```python
from build123d import *

# Parameters (mm, degrees)
SKETCH1_R               = 2.7
BOSS_EXTRUDE1_DEPTH     = 35
CUT_EXTRUDE1_DEPTH      = 36.207669619
CUT_EXTRUDE1_DEPTH_BACK = 36.207669619
SKETCH2_W               = 9
SKETCH2_H               = 0.85
M3_TAPPED_HOLE1_D       = 2.5
M3_TAPPED_HOLE1_DEPTH   = 7.5
M3_TAPPED_HOLE1_TIP     = 0.751075774


with BuildPart() as part:
    # Sketch1 → Boss-Extrude1 (new body)
    with BuildSketch(Plane(origin=(0, 0, 0), x_dir=(0, 0, -1), z_dir=(1, 0, 0))):
        Circle(SKETCH1_R)
    extrude(amount=BOSS_EXTRUDE1_DEPTH)

    # Sketch2 → Cut-Extrude1 (cut, two sides: drawn at the far end of the back side and taken through both)
    with BuildSketch(Plane.XY.offset(-CUT_EXTRUDE1_DEPTH_BACK)):
        with Locations((30.5, 2.275)):
            Rectangle(SKETCH2_W, SKETCH2_H)
        with Locations((30.5, -2.275)):
            Rectangle(SKETCH2_W, SKETCH2_H)
        with Locations((4.5, -2.275)):
            Rectangle(SKETCH2_W, SKETCH2_H)
        with Locations((4.5, 2.275)):
            Rectangle(SKETCH2_W, SKETCH2_H)
    extrude(amount=CUT_EXTRUDE1_DEPTH + CUT_EXTRUDE1_DEPTH_BACK, mode=Mode.SUBTRACT)

    # M3 Tapped Hole1
    with Locations(Plane(origin=(35, 0, 0), x_dir=(0, 0, -1), z_dir=(1, 0, 0))):
        with Locations((0, 0)):
            Hole(M3_TAPPED_HOLE1_D / 2, depth=M3_TAPPED_HOLE1_DEPTH)
            with Locations((0, 0, -(M3_TAPPED_HOLE1_DEPTH + M3_TAPPED_HOLE1_TIP / 2))):  # 118° drill point
                Cone(0, M3_TAPPED_HOLE1_D / 2, M3_TAPPED_HOLE1_TIP, mode=Mode.SUBTRACT)


solid = part.part
```
Source: CAD feature listing. Evaluate the final solid. Frame: model axes, mm. A direction names the side the tool comes from. Round coordinates to 2 decimals unless told otherwise and drop trailing zeros. Loops run counter-clockwise (first coordinate to the right, second up) from the corner with the lowest first, then second, coordinate; pieces in that order, holes last.
(1) Pull-direction query (Y, two-part tool) for faces 4 (the flat face through (30, -1.85, 0)), 5 (the flat face through (26, 2, 0)), 6 (the cylindrical face through (31.2, -1.22, -0.27)); classes: +Y half, -Y half, draft (parallel to the pull), parting line (faces both ways), or undercut.
From the geometry:
face 4: -Y half
face 5: draft
face 6: undercut
(2) Contact query for flat-ended pins moving along their axis: pin 1 Ø3 at (x, z) = (31.5, 0) entering from -Y; pin 2 Ø2 at (x, y) = (15, -2) entering from -Z; pin 3 Ø1.5 at (x, z) = (19, 1.5) entering from -Y. Output: stop coordinate, or through.
From the geometry:
pin 1: stops at y = -1.85
pin 2: stops at z = -2.51
pin 3: stops at y = -2.59
(3) Material intervals for probe 1 along Z at (x, y) = (33, 0); probe 2 along Y at (x, z) = (29, 0.1); probe 3 along Z at (x, y) = (32.5, 0.55), sorted ascending.
From the geometry:
probe 1: z = -2.7 to -1.25, 1.25 to 2.7
probe 2: y = -1.85 to -1.25, 1.25 to 1.85
probe 3: z = -2.64 to -1.12, 1.12 to 2.64
(4) Access query for faces 1 (the flat face through (26, -2, 0)), 2 (the flat face through (4, -1.85, 0)), 3 (the flat face through (4, 1.85, 0)). Directions: +Z, -Z, +X, -X, +Y, -Y. A direction counts if a zero-diameter tool reaches every point of the face in a straight line with its end or side. Return the directions, or none.
From the geometry:
face 1: +Z, -Z, +X, -Y
face 2: +Z, -Z, -X, -Y
face 3: +Z, -Z, -X, +Y
(5) Section query A-A (x = 18). Output: boundary loops of the cut face in (y, z).
From the geometry:
outline: circle Ø5.4 at (0, 0)
